from build123d import *

# Parameters (mm, degrees)
EXTRUDE3_DEPTH    = 2.54
CIRPATTERN1_COUNT = 6
FILLET4_R         = 0.127
LPATTERN1_COUNT   = 5
LPATTERN1_PITCH   = 0.4572


with BuildPart() as part:
    # Sketch1 → Revolve1 (revolve)
    with BuildSketch(Plane(origin=(0, 0, 0), x_dir=(1, 0, 0), z_dir=(0, 1, 0)), mode=Mode.PRIVATE) as revolve1_sk:
        Polygon((23.876, 2.032), (31.242, 2.032), (35.814, 0.367928089), (35.12539449, -1.524), (30.55339449, 0.140071911), (23.876, 0.140071911), align=None)
    revolve(revolve1_sk.sketch.rotate(Axis((0, 0, -37.83814433), (0, 0, 1)), 180), axis=Axis((0, 0, -37.83814433), (0, 0, 1)))  # turned: the seam where the file's is

    # Sketch3 → Extrude3 (add, symmetric)
    with BuildSketch(Plane(origin=(0, 0, 0), x_dir=(1, 0, 0), z_dir=(0, 1, 0))):
        Polygon((34.798, 0.737721847), (37.423501182, -0.217882434), (36.734895673, -2.109810522), (34.10939449, -1.154206242), align=None)
    extrude3 = extrude(amount=EXTRUDE3_DEPTH, both=True)

    # CirPattern1: Extrude3 ×6 about axis
    cirpattern1_axis = Axis((0, 0, 0), (0, 0, 1))
    for i in range(1, CIRPATTERN1_COUNT):
        add(extrude3.rotate(cirpattern1_axis, i * 360 / CIRPATTERN1_COUNT))

    # Fillet4
    fillet4_edges = [part.edges().sort_by_distance(p)[0] for p in [
        (23.876, 0, -0.140071911),
        (23.876, 0, -2.032),
    ]]
    fillet(fillet4_edges, radius=FILLET4_R)

    # Sketch4 → Cut-Revolve1 (revolve, cut)
    with BuildSketch(Plane(origin=(0, 0, 0), x_dir=(1, 0, 0), z_dir=(0, 1, 0))):
        Polygon((-23.876, 0.140071911), (-23.876, 1.019953721), (-24.638, 0.580012816), align=None)
    cut_revolve1 = revolve(axis=Axis((0, 0, -37.83814433), (0, 0, 1)), mode=Mode.SUBTRACT)

    # LPattern1: Cut-Revolve1 ×5
    with Locations(*[(0, 0, -i * LPATTERN1_PITCH) for i in range(1, LPATTERN1_COUNT)]):
        add(cut_revolve1, mode=Mode.SUBTRACT)


solid = part.part
Part model, mm, in its own coordinate system. A direction names the side the tool comes from. Coordinates: 2 decimals unless noted, no trailing zeros. Loops run counter-clockwise (first coordinate to the right, second up) from the corner with the lowest first, then second, coordinate; pieces in that order, holes last. Notation, with made-up numbers: (22.5, -13.5) - (70.5, -13.5) arc R30 ccw to (70.5, 10.5) - close; hole circle Ø2 at (37, -29.75). An arc over 180 degrees is marked (long way). Write each question's results on one line, items separated by ' | '. Start each with the question number.
Q1. Which spindle directions (+Z, -Z, +X, -X, +Y, -Y) get a long thin tool onto all of the face, cutting with end or side? Do faces 1 (the flat face through (-18.077, 31.239, -0.267)), 2 (the flat face through (-13.4, 20.2, -0.14)). Say none if no direction does.
Q2. Slice it at A-A on x = 0. Give the cut face in (y, z).
Q3. Probe line 1 along Y through (x, z) = (-3, -0.2); line 2 along Z through (x, y) = (14, -26); line 3 along Y through (x, z) = (15.5, -0.3). List the from-to ranges inside material, lowest first.
Q4. Drop flat-ended pins along their axis: pin 1 Ø4 at (x, y) = (27, -9.5) entering from +Z; pin 2 Ø1 at (x, z) = (1.5, 0.5) entering from -Y; pin 3 Ø1.5 at (y, z) = (-18.5, -0.5) entering from +X; pin 4 Ø1 at (x, y) = (-5.5, 21) entering from -Z. Give the stop position or say it passes through.
Q5. Two-plate mould, pull along Y, no slides. Class faces 3 (the flat face through (-20.26, 30.01, 0.98)), 4 (the flat face through (-37.084, -0.036, 1.151)), 5 (the flat face through (15.86, -32.55, 0.98)): +Y half, -Y half, draft (parallel to the pull), parting line (faces both ways), or undercut.
Answer:
1) face 1: -Z, -X, +Y | face 2: +Z
2) outline: (-35.81, -0.37) - (-31.24, -2.03) - (-24.5, -2.03) - (-24.64, -1.95) - (-24.24, -1.72) - (-24.64, -1.49) - (-24.24, -1.27) - (-24.64, -1.04) - (-24.24, -0.81) - (-24.64, -0.58) - (-23.92, -0.17) arc R0.13 ccw to (-24, -0.14) - (-30.55, -0.14) - (-35.13, 1.52) - close; (23.92, -0.17) - (24.64, -0.58) - (24.24, -0.81) - (24.64, -1.04) - (24.24, -1.27) - (24.64, -1.49) - (24.24, -1.72) - (24.64, -1.95) - (24.5, -2.03) - (31.24, -2.03) - (35.81, -0.37) - (35.13, 1.52) - (30.55, -0.14) - (24, -0.14) arc R0.13 ccw to start
3) line 1: y = -35.63 to -23.79, 23.79 to 35.63 | line 2: z = -2.03 to -0.14 | line 3: y = -32.26 to -18.52, 18.52 to 32.26
4) pin 1: stops at z = -0.11 | pin 2: stops at y = -35.65 | pin 3: stops at x = 31.1 | pin 4: passes through
5) face 3: undercut | face 4: draft | face 5: -Y half
